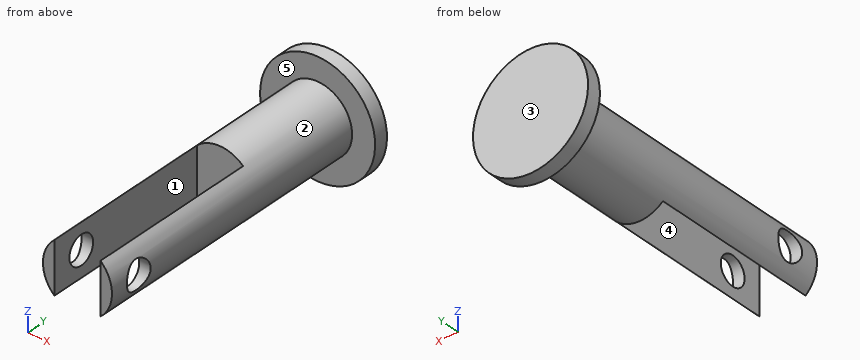
from build123d import *

# Parameters (mm, degrees)
SKETCH_4_W          = 16
SKETCH_4_H          = 70
CUT_EXTRUDE_1_DEPTH = 15
SKETCH_6_R          = 5
CUT_EXTRUDE_2_DEPTH = 15


with BuildPart() as part:
    # 草图1 → 旋转1 (revolve)
    with BuildSketch(Plane.XY, mode=Mode.PRIVATE) as revolve_1_sk:
        Polygon((-0.455930312, 112.0664832), (19.544069688, 112.0664832), (19.544069688, 107.0664832), (11.544069688, 107.0664832), (11.544069688, 6.0664832), (-0.455930312, 6.0664832), align=None)
    revolve(revolve_1_sk.sketch.rotate(Axis((-0.455930312, 6.0664832, 0), (0, 1, 0)), 90), axis=Axis((-0.455930312, 6.0664832, 0), (0, 1, 0)))

    # 草图4 → 切除-拉伸1 (cut, symmetric)
    with BuildSketch(Plane.XY):
        with Locations((-0.455930312, 31.0664832)):
            Rectangle(SKETCH_4_W, SKETCH_4_H)
    extrude(amount=CUT_EXTRUDE_1_DEPTH, both=True, mode=Mode.SUBTRACT)

    # 草图6 → 切除-拉伸2 (cut, symmetric)
    with BuildSketch(Plane(origin=(0, 0, 0), x_dir=(0, 0, -1), z_dir=(1, 0, 0))):
        with Locations((0, 17.347075097)):
            Circle(SKETCH_6_R)
    extrude(amount=CUT_EXTRUDE_2_DEPTH, both=True, mode=Mode.SUBTRACT)


solid = part.part
Input: part model. Units: mm. Frame: model coordinates. Face numbers are marked on the shaded views. A direction names the side the tool comes from. Give positions to 0.01 mm unless a question says otherwise; leave off trailing zeros. Order: outer loops, then holes, each group sorted by start corner. A loop starts at its lowest first (then second) coordinate and runs counter-clockwise, first axis right, second up.
Q1. Ray query, probe 1 along Y at (x, z) = (-10.35, 0); probe 2 along Y at (x, z) = (0, -2); probe 3 along Y at (x, z) = (-10, 9). Return the intervals inside material, ascending.
Checked values:
probe 1: y = 6.07 to 12.35, 22.35 to 112.07
probe 2: y = 66.07 to 112.07
probe 3: y = 107.07 to 112.07
Q2. Contact query for flat-ended pins moving along their axis: pin 1 Ø10 at (x, y) = (5.5, 63.5) entering from -Z; pin 2 Ø8 at (x, y) = (5.5, 80) entering from +Z; pin 3 Ø19.5 at (y, z) = (35.5, -4.5) entering from +X. Output: stop coordinate, or through.
Checked values:
pin 1: stops at z = -11.88
pin 2: stops at z = 11.84
pin 3: stops at x = 11.54
Q3. Section C-C on y = 61. Output: boundary loops of the cut face in (x, z).
Checked values:
outline: (-8.46, -8.94) - (-8.46, 8.94) arc R12 ccw to start; (7.54, -8.94) arc R12 ccw to (7.54, 8.94) - close
Q4. Draft query along X for the marked faces 1, 2 and 3. Return one class per face: +X half, -X half, draft (parallel to the pull), parting line (faces both ways), or undercut.
Checked values:
face 1: undercut
face 2: parting line
face 3: draft
Q5. Section D-D on z = -7.5. Output: boundary loops of the cut face in (x, y), and give its area (3 significant figures).
Checked values:
outline: (-19, 107.07) - (-9.82, 107.07) - (-9.82, 6.07) - (-8.46, 6.07) - (-8.46, 66.07) - (7.54, 66.07) - (7.54, 6.07) - (8.91, 6.07) - (8.91, 107.07) - (18.08, 107.07) - (18.08, 112.07) - (-19, 112.07) - close
area: 1,120 mm2
Q6. Set-up query: the marked faces 4 and 5. Return all of +Z, -Z, +X, -X, +Y, -Y with unobstructed straight access to the full face (end or side cutting, diameter ignored); none if empty.
Checked values:
face 4: +Z, -Z, -Y
face 5: -Y
Q7. Section B-B on x = -5.5. Output: boundary loops of the cut face in (y, z).
Checked values:
outline: (66.07, -10.89) - (107.07, -10.89) - (107.07, -19.35) - (112.07, -19.35) - (112.07, 19.35) - (107.07, 19.35) - (107.07, 10.89) - (66.07, 10.89) - close
Q8. Section A-A on z = 0. Output: boundary loops of the cut face in (x, y).
Checked values:
outline: (-20.46, 107.07) - (-12.46, 107.07) - (-12.46, 22.35) - (-8.46, 22.35) - (-8.46, 66.07) - (7.54, 66.07) - (7.54, 22.35) - (11.54, 22.35) - (11.54, 107.07) - (19.54, 107.07) - (19.54, 112.07) - (-20.46, 112.07) - close; (-12.46, 6.07) - (-8.46, 6.07) - (-8.46, 12.35) - (-12.46, 12.35) - close; (7.54, 6.07) - (11.54, 6.07) - (11.54, 12.35) - (7.54, 12.35) - close
